The figure shows three views and two pictorial views of one solid part (mm, origin at its lowest corner). Answer the questions. Coordinates: 2 decimals unless noted, no trailing zeros. Loops run counter-clockwise (first coordinate to the right, second up) from the corner with the lowest first, then second, coordinate; pieces in that order, holes last. Notation, with made-up numbers: (52.25, 84.5) -> (80.25, 84.5) arc R20 ccw to (80.25, 104.5) -> close; hole circle Ø4 at (-3.75, 27). An arc over 180 degrees is marked (long way). Answer in a Markdown table with one row per item.
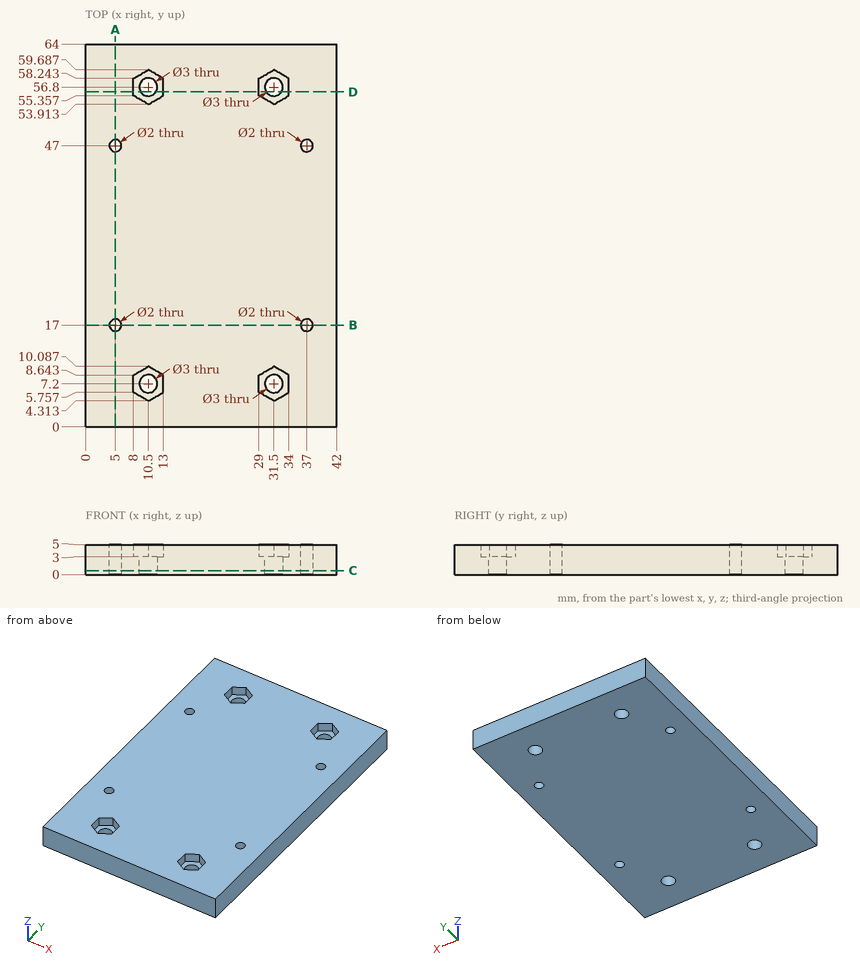
Item 1: A cutting plane is placed at D-D, the plane y = 56. Determine the outline of the cut face in (x, z).
Findings below:
| item | result |
|---|---|
| outline | (0, 0) -> (9.23, 0) -> (9.23, 3) -> (8, 3) -> (8, 5) -> (0, 5) -> close; (11.77, 0) -> (30.23, 0) -> (30.23, 3) -> (29, 3) -> (29, 5) -> (13, 5) -> (13, 3) -> (11.77, 3) -> close; (32.77, 0) -> (42, 0) -> (42, 5) -> (34, 5) -> (34, 3) -> (32.77, 3) -> close |
Item 2: A cutting plane is placed at B-B, the plane y = 17. Determine the outline of the cut face in (x, z), plus the area to 3 significant figures.
Findings below:
| item | result |
|---|---|
| outline | (0, 0) -> (4, 0) -> (4, 5) -> (0, 5) -> close; (6, 0) -> (36, 0) -> (36, 5) -> (6, 5) -> close; (38, 0) -> (42, 0) -> (42, 5) -> (38, 5) -> close |
| area | 190 mm2 |
Item 3: A flat-ended cylindrical pin translates along its axis: pin 1 Ø4 at (x, y) = (31.5, 7.2) entering from +Z. Find the tip coordinate at first contact, or state that the pin passes through.
Findings below:
| item | result |
|---|---|
| pin 1 | stops at z = 3 |
Item 4: A cutting plane is placed at A-A, the plane x = 5. Determine the outline of the cut face in (y, z), plus the area to 3 significant figures.
Findings below:
| item | result |
|---|---|
| outline | (0, 0) -> (16, 0) -> (16, 5) -> (0, 5) -> close; (18, 0) -> (46, 0) -> (46, 5) -> (18, 5) -> close; (48, 0) -> (64, 0) -> (64, 5) -> (48, 5) -> close |
| area | 300 mm2 |
Item 5: Find the intervals of material crossed by probe 1 along Y at (x, z) = (31.5, 1.5); probe 2 along Y at (x, z) = (37, 2.2); probe 3 along X at (y, z) = (56.8, 1.2), in increasing order.
Findings below:
| item | result |
|---|---|
| probe 1 | y = 0 to 5.7, 8.7 to 55.3, 58.3 to 64 |
| probe 2 | y = 0 to 16, 18 to 46, 48 to 64 |
| probe 3 | x = 0 to 9, 12 to 30, 33 to 42 |
Item 6: A cutting plane is placed at C-C, the plane z = 0.7. Count the separate pieces of the cut face and the enclosed holes in it, plus the area to 3 significant figures.
Findings below:
| item | result |
|---|---|
| separate pieces | 1 |
| enclosed holes | 8 |
| area | 2,650 mm2 |
